Read the model definition and answer for the solid it produces. Units are mm, in the model's axes. A direction names the side the tool comes from. Coordinates: 2 decimals unless noted, no trailing zeros. Write each loop counter-clockwise with the first axis right and the second up, starting at its lowest first coordinate (ties: lowest second). Pieces come first, ordered by that corner, then holes.
(1) Which of the six approach directions +Z, -Z, +X, -X, +Y, -Y give full straight-line access (tool end or side, diameter ignored) to faces 1 (the flat face through (0, 7.5, 0)), 2 (the cylindrical face through (1.617, 1.232, -0.67)), 3 (the flat face through (-3.1, 2.5, 0.2)), 4 (the flat face through (3.1, 2.5, -0.2))?
(2) Section C-C on y = 0.5 is taken. Write down the section's boundary in (x, z), then the cut area to 3 significant figures.
(3) Section B-B on z = 0 is taken. Write down the section's boundary in (x, y), then the cut area to 3 significant figures.
(4) Find the intervals of material crossed by probe 1 along Z at (x, y) = (0, 2.05); probe 2 along Z at (x, y) = (1.5, 1.5), in increasing order.
(5) Given pin 1 (1.5 mm diameter, centred on x = -2.5, y = 1, fed in from -Z), flat-ended and moving along its own axis, determine where the tip first touches the part or whether it passes through.
(6) Section A-A on y = 5.5 is taken. Write down the section's boundary in (x, z).
from build123d import *

# Parameters (mm, degrees)
SKETCH1_R           = 2.95
BOSS_EXTRUDE1_DEPTH = 2.5
SKETCH2_R           = 1.75
CUT_EXTRUDE1_DEPTH  = 2.5
SKETCH3_W           = 6.9
SKETCH3_H           = 5.9
BOSS_EXTRUDE2_DEPTH = 5
FILLET1_R           = 2.54
FILLET2_R           = 0.75


with BuildPart() as part:
    # Sketch1 → Boss-Extrude1 (new body)
    with BuildSketch(Plane(origin=(0, 0, 0), x_dir=(1, 0, 0), z_dir=(0, 1, 0))):
        Circle(SKETCH1_R)
    extrude(amount=BOSS_EXTRUDE1_DEPTH)

    # Sketch2 → Cut-Extrude1 (cut)
    with BuildSketch(Plane.XZ):
        Circle(SKETCH2_R)
    extrude(amount=-CUT_EXTRUDE1_DEPTH, mode=Mode.SUBTRACT)

    # Sketch3 → Boss-Extrude2 (add)
    with BuildSketch(Plane(origin=(0, 2.5, 0), x_dir=(1, 0, 0), z_dir=(0, 1, 0))):
        Rectangle(SKETCH3_W, SKETCH3_H)
    extrude(amount=BOSS_EXTRUDE2_DEPTH)

    # Fillet1
    fillet1_edges = [part.edges().sort_by_distance(p)[0] for p in [
        (3.45, 5, 2.95),
        (3.45, 5, -2.95),
        (-3.45, 5, -2.95),
        (-3.45, 5, 2.95),
    ]]
    fillet(fillet1_edges, radius=FILLET1_R)

    # Fillet2
    fillet2_edges = [part.edges().sort_by_distance(p)[0] for p in [
        (-3.45, 7.5, 0),
        (0, 7.5, -2.95),
        (3.45, 7.5, 0),
        (0, 7.5, 2.95),
        (-2.706051224, 7.5, 2.206051224),
        (2.706051224, 7.5, 2.206051224),
        (2.706051224, 7.5, -2.206051224),
        (-2.706051224, 7.5, -2.206051224),
    ]]
    fillet(fillet2_edges, radius=FILLET2_R)


solid = part.part
Response:
1. face 1: +Z, -Z, +X, -X, +Y
1. face 2: -Y
1. face 3: -X, -Y
1. face 4: +X, -Y
2. outline: circle Ø5.9 at (0, 0); hole circle Ø3.5 at (0, 0)
2. area: 17.7 mm2
3. outline: (-3.45, 2.5) - (-2.95, 2.5) - (-2.95, 0) - (-1.75, 0) - (-1.75, 2.5) - (1.75, 2.5) - (1.75, 0) - (2.95, 0) - (2.95, 2.5) - (3.45, 2.5) - (3.45, 6.75) arc R0.75 ccw to (2.7, 7.5) - (-2.7, 7.5) arc R0.75 ccw to (-3.45, 6.75) - close
3. area: 40.3 mm2
4. probe 1: z = -2.95 to -1.75, 1.75 to 2.95
4. probe 2: z = -2.54 to -0.9, 0.9 to 2.54
5. pin 1: stops at z = -2.37
6. outline: (-3.45, -0.41) arc R2.54 ccw to (-0.91, -2.95) - (0.91, -2.95) arc R2.54 ccw to (3.45, -0.41) - (3.45, 0.41) arc R2.54 ccw to (0.91, 2.95) - (-0.91, 2.95) arc R2.54 ccw to (-3.45, 0.41) - close
